```python
from build123d import *

# Parameters (mm, degrees)
SKETCH1_R           = 12
BOSS_EXTRUDE1_DEPTH = 30
SKETCH2_R           = 8
BOSS_EXTRUDE2_DEPTH = 5
SKETCH4_R           = 1.579295677
CUT_EXTRUDE3_DEPTH  = 3
SKETCH5_R           = 3
BOSS_EXTRUDE3_DEPTH = 10
SKETCH6_R           = 8.773986351
BOSS_EXTRUDE4_DEPTH = 3
FILLET1_R           = 2


with BuildPart() as part:
    # Sketch1 → Boss-Extrude1 (new body)
    with BuildSketch(Plane.XY):
        with Locations((5.178689325, -6.92509434)):
            Circle(SKETCH1_R)
    extrude(amount=BOSS_EXTRUDE1_DEPTH)

    # Sketch2 → Boss-Extrude2 (add)
    with BuildSketch(Plane.XY.offset(30)):
        with Locations((5.178689325, -6.92509434)):
            Circle(SKETCH2_R)
    extrude(amount=BOSS_EXTRUDE2_DEPTH)

    # Sketch4 → Cut-Extrude3 (cut)
    with BuildSketch(Plane.XY.offset(35)):
        with Locations((5.178689325, 2.995609984)):
            Circle(SKETCH4_R)
        with Locations((15.099393648, -6.92509434)):
            Circle(SKETCH4_R)
        with Locations((5.178689325, -16.845798663)):
            Circle(SKETCH4_R)
        with Locations((-4.742014998, -6.92509434)):
            Circle(SKETCH4_R)
    extrude(amount=-CUT_EXTRUDE3_DEPTH, mode=Mode.SUBTRACT)

    # Sketch5 → Boss-Extrude3 (add)
    with BuildSketch(Plane.XY.offset(35)):
        with Locations((5.178689325, -6.92509434)):
            Circle(SKETCH5_R)
    extrude(amount=BOSS_EXTRUDE3_DEPTH)

    # Sketch6 → Boss-Extrude4 (add)
    with BuildSketch(Plane(origin=(0, 0, 0), x_dir=(-1, 0, 0), z_dir=(0, 0, -1))):
        with Locations((-5.178689325, -6.92509434)):
            Circle(SKETCH6_R)
    extrude(amount=BOSS_EXTRUDE4_DEPTH)

    # Fillet1
    fillet1_edges = [part.edges().sort_by_distance(p)[0] for p in [
        (-6.821310675, -6.92509434, 0),
    ]]
    fillet(fillet1_edges, radius=FILLET1_R)


solid = part.part
```
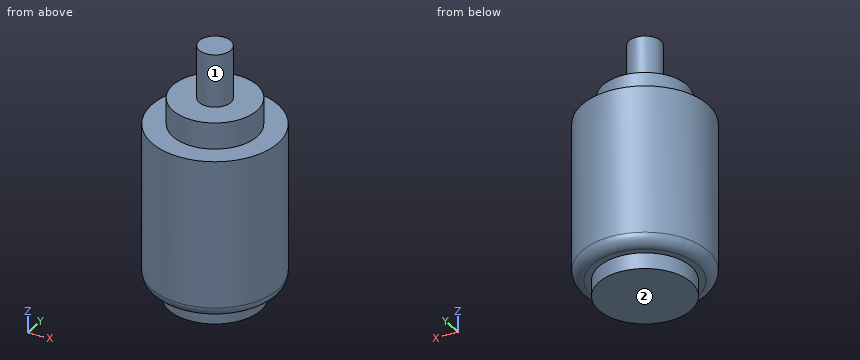
Can you work these out from the model? Positions are in its coordinate system, mm. Face numbers are marked on the shaded views. A direction names the side the tool comes from. Round coordinates to 2 decimals unless told otherwise and drop trailing zeros. Loops run counter-clockwise (first coordinate to the right, second up) from the corner with the lowest first, then second, coordinate; pieces in that order, holes last. Notation, with made-up numbers: (-32.75, -15.75) -> (-16.75, -15.75) arc R10 cw to (-16.75, -5.75) -> close; hole circle Ø5 at (-14, 66). An arc over 180 degrees is marked (long way). One line per item, written item: value. Start each with the question number.
1. If we section it at B-B, the plane z = 36.5: Write out the boundary of the cut face in (x, y).
2. For the marked faces 1 and 2, which set-ups out of +Z, -Z, +X, -X, +Y, -Y let a thin tool reach every point of the face, with its end or its side?
3. If I drill on probe 1 along Z at (x, y) = (4.5, -2.5); probe 2 along Y at (x, z) = (5.25, 18.5); probe 3 along Z at (x, y) = (13.75, -14.25), over which ranges is the centre line in solid material (lowest first)?
4. If we section it at A-A, the plane z = 21.5: Write out the boundary of the cut face in (x, y), then the cut area to 3 significant figures.
5. For pin 1 (1.5 mm diameter, centred on y = -3.5, z = 40, fed in from -X); pin 2 (8 mm diameter, centred on x = 11, z = 38, fed in from +Y); pin 3 (5 mm diameter, centred on x = 11.5, z = 3.5, fed in from -Y), each with a flat end and sliding along its axis, tell me the tip position at first contact or that it passes through.
Calculated:
1. outline: circle Ø6 at (5.18, -6.93)
2. face 1: +Z
2. face 2: -Z, +X, -X, +Y, -Y
3. probe 1: z = -3 to 35
3. probe 2: y = -18.92 to 5.07
3. probe 3: z = 0.46 to 30
4. outline: circle Ø24 at (5.18, -6.93)
4. area: 452 mm²
5. pin 1: stops at x = 3.82
5. pin 2: stops at y = 0.42
5. pin 3: stops at y = -18.3
